```python
from build123d import *

# Parameters (mm, degrees)
BOSS_EXTRU_1_DEPTH      = 10
ENL_V_MAT_EXTRU_1_DEPTH = 90.16782474
ESQUISSE3_R             = 2
ENL_V_MAT_EXTRU_2_DEPTH = 90.167824766
ENL_V_MAT_EXTRU_3_DEPTH = 3.3
ENL_V_MAT_EXTRU_4_DEPTH = 102.195391925


with BuildPart() as part:
    # Esquisse1 → Boss.-Extru.1 (new body)
    with BuildSketch(Plane(origin=(0, 0, 0), x_dir=(0, 0, -1), z_dir=(1, 0, 0))):
        with BuildLine():
            Line((-87.523995303, -46.245048312), (-87.523995303, -38.999770184))
            ThreePointArc((-87.523995303, -38.999770184), (-86.645315647, -36.87844984), (-84.523995303, -35.999770184))
            Line((-84.523995303, -35.999770184), (-70.36921968, -35.999770184))
            ThreePointArc((-70.36921968, -35.999770184), (-60.503302019, -39.700935345), (-50.637384358, -35.999770184))
            Line((-50.637384358, -35.999770184), (-32.848182024, -35.999770184))
            Line((-32.848182024, -35.999770184), (-32.848182024, -44.534320741))
            ThreePointArc((-32.848182024, -44.534320741), (-33.712584856, -46.641267521), (-35.80766518, -47.534047126))
            Line((-35.80766518, -47.534047126), (-78.000260647, -48.103936043))
            ThreePointArc((-78.000260647, -48.103936043), (-81.919367341, -49.773558375), (-86.070253365, -48.815862581))
            ThreePointArc((-86.070253365, -48.815862581), (-87.135390925, -47.72173816), (-87.523995303, -46.245048312))
        make_face()
    extrude(amount=BOSS_EXTRU_1_DEPTH)

    # Esquisse2 → Enlèv. mat.-Extru.1 (cut, through all)
    with BuildSketch(Plane(origin=(0, -35.999770184, 0), x_dir=(1, 0, 0), z_dir=(0, 1, 0))):
        with BuildLine():
            Line((3, -82.523995303), (3, -81.523995303))
            ThreePointArc((3, -81.523995303), (5, -79.523995303), (7, -81.523995303))
            Line((7, -81.523995303), (7, -82.523995303))
            ThreePointArc((7, -82.523995303), (5, -84.523995303), (3, -82.523995303))
        make_face()
    extrude(amount=-ENL_V_MAT_EXTRU_1_DEPTH, mode=Mode.SUBTRACT)

    # Esquisse3 → Enlèv. mat.-Extru.2 (cut, through all)
    with BuildSketch(Plane(origin=(0, -35.999770184, 0), x_dir=(1, 0, 0), z_dir=(0, 1, 0))):
        with Locations(Location((5, -37.848182024, 0), (0, 0, 270))):
            Circle(ESQUISSE3_R)
    extrude(amount=-ENL_V_MAT_EXTRU_2_DEPTH, mode=Mode.SUBTRACT)

    # Esquisse4 → Enlèv. mat.-Extru.3 (cut)
    with BuildSketch(Plane(origin=(0, -47.999770184, 141.218220364), x_dir=(1, 0, 0), z_dir=(0, 1, 0))):
        Polygon((5, 107.552964167), (1.377479972, 105.461501254), (1.377479972, 101.278575427), (5, 99.187112513), (8.622520028, 101.278575427), (8.622520028, 105.461501254), align=None)
    extrude(amount=ENL_V_MAT_EXTRU_3_DEPTH, mode=Mode.SUBTRACT)

    # Esquisse5 → Enlèv. mat.-Extru.4 (cut, through all)
    with BuildSketch(Plane(origin=(10, 0, 0), x_dir=(0, 0, -1), z_dir=(1, 0, 0))):
        with BuildLine():
            Line((-70.36921968, -35.999770184), (-71.83186465, -35.999770184))
            ThreePointArc((-71.83186465, -35.999770184), (-60.503302019, -40.700935345), (-49.174739388, -35.999770184))
            Line((-49.174739388, -35.999770184), (-50.637384358, -35.999770184))
            Line((-50.637384358, -35.999770184), (-70.36921968, -35.999770184))
        make_face()
    extrude(amount=-ENL_V_MAT_EXTRU_4_DEPTH, mode=Mode.SUBTRACT)


solid = part.part
```
Build history of the part. All positions in model axes, mm. A direction names the side the tool comes from. Round coordinates to 2 decimals unless told otherwise and drop trailing zeros. Order: outer loops, then holes, each group sorted by start corner. A loop starts at its lowest first (then second) coordinate and runs counter-clockwise, first axis right, second up. Notation, with made-up numbers: (-15.5, 30) - (27.5, 30) arc R22 cw to (27.5, 67) - close; hole circle Ø9 at (-3, 78.25). An arc over 180 degrees is marked (long way). Use a Markdown table: item, result.
1) Saw through at A-A on y = -37.5. Write the cut outline in (x, z).
Recorded:
| item | result |
|---|---|
| outline | (0, 32.85) - (10, 32.85) - (10, 50.9) - (0, 50.9) - close; (0, 70.1) - (10, 70.1) - (10, 87.12) - (0, 87.12) - close; hole circle Ø4 at (5, 37.85); hole (3, 81.52) arc R2 ccw to (7, 81.52) - (7, 82.52) arc R2 ccw to (3, 82.52) - close |
2) Pull direction X, two halves, no side cores. Call faces 1 (the face through (4.93, -47.741, 87.125)), 2 (the face through (3.16, -46.18, 40.97)), 3 (the face through (0, -43, 60)): pulls with the +X half, pulls with the -X half, needs draft (parallel to the pull), parting line crosses it, or undercut.
Recorded:
| item | result |
|---|---|
| face 1 | needs draft |
| face 2 | undercut |
| face 3 | pulls with the -X half |
3) Saw through at B-B on z = 82. Write the cut outline in (x, y), and give its area (3 significant figures).
Recorded:
| item | result |
|---|---|
| outline | (0, -49.78) - (3, -49.78) - (3, -36) - (0, -36) - close; (7, -49.78) - (10, -49.78) - (10, -36) - (7, -36) - close |
| area | 82.7 mm² |
4) Tool access for faces 4 (the face through (8.623, -46, 38)), 5 (the face through (3, -43, 82)), 6 (the face through (5.1, -40.7, 60.7)): list every direction of +Z, -Z, +X, -X, +Y, -Y with a clear straight run to the whole face (end or side of a thin tool).
Recorded:
| item | result |
|---|---|
| face 4 | -Y |
| face 5 | +Y, -Y |
| face 6 | +X, -X, +Y |
5) Saw through at C-C on x = 5.75. Write the cut outline in (y, z).
Recorded:
| item | result |
|---|---|
| outline | (-49.55, 84.38) - (-36, 84.38) - (-36, 84.52) arc R3 ccw to (-39, 87.52) - (-46.25, 87.52) arc R3 ccw to (-48.82, 86.07) arc R6.88 ccw to start; (-49.18, 79.67) arc R6.88 ccw to (-48.1, 78) - (-47.61, 41.6) - (-44.7, 41.6) - (-44.7, 39.7) - (-36, 39.7) - (-36, 49.17) arc R16 cw to (-36, 71.83) - (-36, 79.67) - close; (-46.97, 34.1) arc R3 ccw to (-44.53, 32.85) - (-36, 32.85) - (-36, 35.99) - (-44.7, 35.99) - (-44.7, 34.1) - close |
6) Flat gauge pins, fed straight in: pin 1 Ø5 at (x, z) = (5, 37.85) entering from -Y; pin 2 Ø4 at (x, z) = (6, 56.5) entering from +Y; pin 3 Ø6 at (x, z) = (6.5, 39) entering from -Y. Where does each tip first touch, or does it go through?
Recorded:
| item | result |
|---|---|
| pin 1 | stops at y = -44.7 |
| pin 2 | stops at y = -39.53 |
| pin 3 | stops at y = -47.62 |
7) Wall check: L1, parallel to X at y = -41.75, z = 82; L2, parallel to Z at x = 6, y = -46; L3, parallel to X at y = -47.5, z = 38. Give the ranges that are in metal, low to high.
Recorded:
| item | result |
|---|---|
| L1 | x = 0 to 3, 7 to 10 |
| L2 | z = 33.23 to 34.24, 41.45 to 79.79, 84.26 to 87.52 |
| L3 | x = 0 to 1.38, 8.62 to 10 |
8) Saw through at D-D on z = 54. Write the cut outline in (x, y), and give its area (3 significant figures).
Recorded:
| item | result |
|---|---|
| outline | (0, -47.78) - (10, -47.78) - (10, -39.32) - (0, -39.32) - close |
| area | 84.6 mm² |
